Build history of the part. All positions in model axes, mm. A direction names the side the tool comes from. Round coordinates to 2 decimals unless told otherwise and drop trailing zeros. Loops run counter-clockwise (first coordinate to the right, second up) from the corner with the lowest first, then second, coordinate; pieces in that order, holes last. Notation, with made-up numbers: (-11, -19.75) -> (-6, -19.75) arc R32 cw to (-6, 18.25) -> close; hole circle Ø9 at (53.25, -4.5). An arc over 180 degrees is marked (long way). Put each result on its own line as item: value. Start each with the question number.
Item 1: Flat gauge pins, fed straight in: pin 1 Ø2.5 at (x, z) = (7, 1.5) entering from +Y; pin 2 Ø2 at (y, z) = (32, 2.5) entering from -X. Where does each tip first touch, or does it go through?
Item 2: Cut at A-A, the plane z = 4.5. List the corners of the cut face in (x, y), plus the area to 3 significant figures.
Item 3: Drill centre lines: probe 1 along Y at (x, z) = (-0.25, 4.55); probe 2 along X at (y, z) = (24.5, 3); probe 3 along Y at (x, z) = (-5.5, 4.25). Where is each one in solid material? Low to high. Write a range as [from, to].
Item 4: Cut at B-B, the plane x = -3.75. List the corners of the cut face in (y, z).
Item 5: Pull direction Y, two halves, no side cores. Call faces 5 (the flat face through (-2, 26, 2)), 6 (the flat face through (-1, 26, 5)), 7 (the flat face through (7, 45.691, 2)): +Y half, -Y half, draft (parallel to the pull), parting line (faces both ways), or undercut.
Item 6: Tool access for faces 1 (the flat face through (-7, 45.691, 2)), 2 (the flat face through (6, 42.691, 2)), 3 (the cylindrical face through (-6.35, 5.03, 2.46)), 4 (the flat face through (3.91, 46.68, 2.46)): list every direction of +Z, -Z, +X, -X, +Y, -Y with a clear straight run to the whole face (end or side of a thin tool).
Item 7: Cut at D-D, the plane y = 21.5. List the corners of the cut face in (x, z), plus the area to 3 significant figures.
Item 8: Cut at C-C, the plane y = 3.5. List the corners of the cut face in (x, z), plus the area to 3 significant figures.
```python
from build123d import *

# Parameters (mm, degrees)
F1_DEPTH = 5


with BuildPart() as f1:
    # F0 (on Top) → F1 (new body)
    with BuildSketch(Plane.XY):
        with BuildLine():
            ThreePointArc((2, 4.691482), (4.254997, 2.811583), (5.1, 0))
            Line((5.1, 0), (8.1, 0))
            ThreePointArc((8.1, 0), (6.395702, 4.970412), (2, 7.849204))
            Line((2, 7.849204), (2, 4.691482))
        make_face()
        with BuildLine():
            ThreePointArc((-2, 4.691482), (0, 5.1), (2, 4.691482))
            Line((2, 4.691482), (2, 7.849204))
            ThreePointArc((2, 7.849204), (0, 8.1), (-2, 7.849204))
            Line((-2, 7.849204), (-2, 4.691482))
        make_face()
        with BuildLine():
            ThreePointArc((-5.1, 0), (-4.254997, 2.811583), (-2, 4.691482))
            Line((-2, 4.691482), (-2, 7.849204))
            ThreePointArc((-2, 7.849204), (-6.395702, 4.970412), (-8.1, 0))
            Line((-8.1, 0), (-5.1, 0))
        make_face()
        with BuildLine():
            ThreePointArc((-2, 7.849204), (0, 8.1), (2, 7.849204))
            Line((2, 7.849204), (2, 42.691482))
            Line((2, 42.691482), (-2, 42.691482))
            Line((-2, 42.691482), (-2, 7.849204))
        make_face()
        Polygon((-2, 42.691482), (2, 42.691482), (10, 42.691482), (10, 45.691482), (4.65, 45.691482), (-4.65, 45.691482), (-10, 45.691482), (-10, 42.691482), align=None)
        Polygon((-4.65, 45.691482), (4.65, 45.691482), (3.15, 47.691482), (-3.15, 47.691482), align=None)
    extrude(amount=F1_DEPTH)


solid = f1.part
```
Reply:
1. pin 1: stops at y = 45.69
1. pin 2: stops at x = -2
2. outline: (-10, 42.69) -> (-2, 42.69) -> (-2, 7.85) arc R8.1 ccw to (-8.1, 0) -> (-5.1, 0) arc R5.1 cw to (-2, 4.69) arc R5.1 cw to (2, 4.69) arc R5.1 cw to (5.1, 0) -> (8.1, 0) arc R8.1 ccw to (2, 7.85) -> (2, 42.69) -> (10, 42.69) -> (10, 45.69) -> (4.65, 45.69) -> (3.15, 47.69) -> (-3.15, 47.69) -> (-4.65, 45.69) -> (-10, 45.69) -> close
2. area: 277 mm^2
3. probe 1: y = [5.09, 47.69]
3. probe 2: x = [-2, 2]
3. probe 3: y = [0, 5.95], [42.69, 45.69]
4. outline: (3.46, 0) -> (7.18, 0) -> (7.18, 5) -> (3.46, 5) -> close; (42.69, 0) -> (46.89, 0) -> (46.89, 5) -> (42.69, 5) -> close
5. face 5: undercut
5. face 6: draft
5. face 7: +Y half
6. face 1: +Z, -Z, -X, +Y
6. face 2: +Z, -Z, +X
6. face 3: +Z, -Z, -X
6. face 4: +Z, -Z, +X, +Y
7. outline: (-2, 0) -> (2, 0) -> (2, 5) -> (-2, 5) -> close
7. area: 20.0 mm^2
8. outline: (-7.3, 0) -> (-3.71, 0) -> (-3.71, 5) -> (-7.3, 5) -> close; (3.71, 0) -> (7.3, 0) -> (7.3, 5) -> (3.71, 5) -> close
8. area: 36.0 mm^2
